Job drawing, mm, ordinate dimensions from the low corner. One solid piece. Coordinates: 2 decimals unless noted, no trailing zeros. Order: outer loops, then holes, each group sorted by start corner. A loop starts at its lowest first (then second) coordinate and runs counter-clockwise, first axis right, second up. Notation, with made-up numbers: (73.5, 68.5) - (108.5, 68.5) arc R32 cw to (108.5, 99.5) - close; hole circle Ø9 at (8, -39.75). An arc over 180 degrees is marked (long way). Use a Markdown table: item, result. Add a question column.
1) Saw through at C-C on z = 2. List the corners of the cut face in (x, y), then the cut area to 3 significant figures.
2) Saw through at A-A on y = 23. List the corners of the cut face in (x, z), then the cut area to 3 significant figures.
3) Drop flat-ended pins along their axis: P1, Ø3, axis at x = 15, y = 32.5, coming from the -Z side; P2, Ø1.5, axis at y = 22.5, z = 2, coming from the +X side; P3, Ø1.5, axis at x = 33, z = 2, coming from the -Y side; P4, Ø0.9, axis at y = 17.5, z = 1, coming from the -X side. Give the stop position or say it passes through.
4) Saw through at B-B on x = 38.5. List the corners of the cut face in (y, z).
5) Wall check: L1, parallel to X at y = 2.5, z = 1.1; L2, parallel to X at y = 18.5, z = 1.2; L3, parallel to Y at x = 32.5, z = 0.55. Give the ranges that are in metal, low to high. Write a range as [from, to].
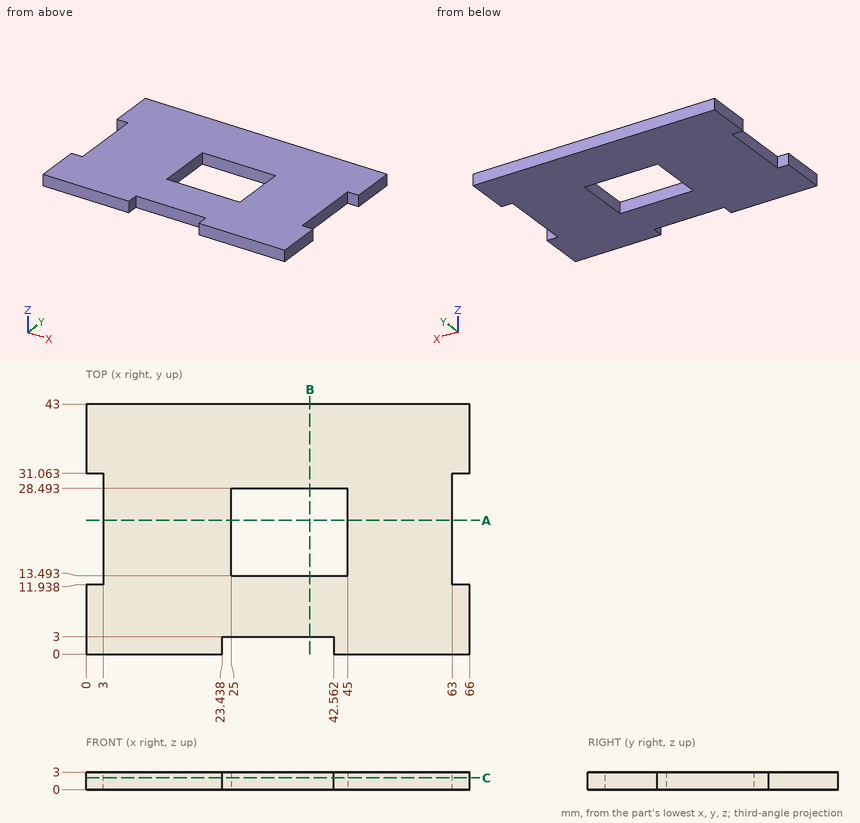
Results are:
| question | item | result |
|---|---|---|
| 1 | outline | (0, 0) - (23.44, 0) - (23.44, 3) - (42.56, 3) - (42.56, 0) - (66, 0) - (66, 11.94) - (63, 11.94) - (63, 31.06) - (66, 31.06) - (66, 43) - (0, 43) - (0, 31.06) - (3, 31.06) - (3, 11.94) - (0, 11.94) - close; hole (25, 13.49) - (45, 13.49) - (45, 28.49) - (25, 28.49) - close |
| 1 | area | 2,370 mm2 |
| 2 | outline | (3, 0) - (25, 0) - (25, 3) - (3, 3) - close; (45, 0) - (63, 0) - (63, 3) - (45, 3) - close |
| 2 | area | 120 mm2 |
| 3 | P1 | z = 0 |
| 3 | P2 | x = 63 |
| 3 | P3 | y = 3 |
| 3 | P4 | x = 3 |
| 4 | outline | (3, 0) - (13.49, 0) - (13.49, 3) - (3, 3) - close; (28.49, 0) - (43, 0) - (43, 3) - (28.49, 3) - close |
| 5 | L1 | [0, 23.44], [42.56, 66] |
| 5 | L2 | [3, 25], [45, 63] |
| 5 | L3 | [3, 13.49], [28.49, 43] |
